The figure shows three views and two pictorial views of one solid part (mm, origin at its lowest corner). Answer the questions. Round coordinates to 2 decimals unless told otherwise and drop trailing zeros. Loops run counter-clockwise (first coordinate to the right, second up) from the corner with the lowest first, then second, coordinate; pieces in that order, holes last. Notation, with made-up numbers: (73.25, 54.25) -> (110.25, 54.25) arc R31 cw to (110.25, 91.25) -> close; hole circle Ø9 at (31, 2.25). An arc over 180 degrees is marked (long way). Write each question's results on one line, items separated by ' | '. Start each with the question number.
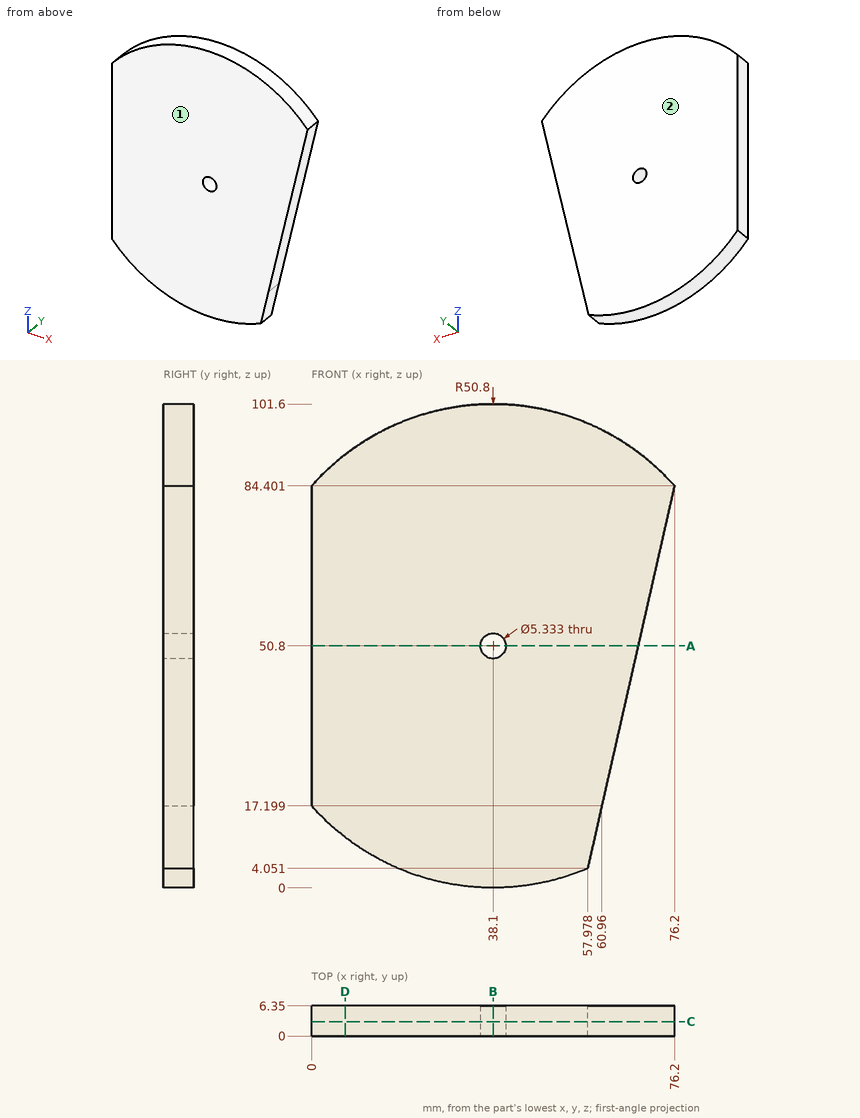
Item 1: The part is cut by section B-B, the plane x = 38.1. Give the vertices of the cut face in (y, z).
Item 2: The part is cut by section D-D, the plane x = 7. Give the vertices of the cut face in (y, z).
Item 3: Determine the mould class of the marked faces 1 and 2 for opening direction Y: +Y half, -Y half, draft (parallel to the pull), parting line (faces both ways), or undercut.
Item 4: The part is cut by section A-A, the plane z = 50.8. Give the vertices of the cut face in (x, y), plus the area to 3 significant figures.
Item 5: Each of these flat-tipped pins is pushed along its axis until it touches: pin 1 Ø8 at (x, z) = (67.5, 33.5) entering from -Y; pin 2 Ø2 at (x, y) = (40, 5.5) entering from -Z; pin 3 Ø2 at (y, z) = (4.5, 22.5) entering from +X. Where does it stop, or does it pass through?
Item 6: Straight lines are drawn through the part: L1, parallel to X at y = 1.75, z = 52.5 (1 decimal); L2, parallel to X at y = 2, z = 50.8; L3, parallel to Z at x = 8, y = 5.75. For each, find the intervals that lie inside material, in ascending order. Write a range as [from, to].
Item 7: The part is cut by section C-C, the plane y = 3. Give the vertices of the cut face in (x, z), plus the area to 3 significant figures.
Report:
1) outline: (0, 0) -> (6.35, 0) -> (6.35, 48.13) -> (0, 48.13) -> close; (0, 53.47) -> (6.35, 53.47) -> (6.35, 101.6) -> (0, 101.6) -> close
2) outline: (0, 10.63) -> (6.35, 10.63) -> (6.35, 90.97) -> (0, 90.97) -> close
3) face 1: -Y half | face 2: +Y half
4) outline: (0, 0) -> (35.43, 0) -> (35.43, 6.35) -> (0, 6.35) -> close; (40.77, 0) -> (68.58, 0) -> (68.58, 6.35) -> (40.77, 6.35) -> close | area: 402 mm2
5) pin 1: stops at y = 0 | pin 2: stops at z = 0.01 | pin 3: stops at x = 62.39
6) L1: x = [0, 36], [40.2, 69] | L2: x = [0, 35.43], [40.77, 68.58] | L3: z = [9.88, 91.72]
7) outline: (0, 17.2) arc R50.8 ccw to (57.98, 4.05) -> (76.2, 84.4) arc R50.8 ccw to (0, 84.4) -> close; hole circle Ø5.33 at (38.1, 50.8) | area: 6,280 mm2
